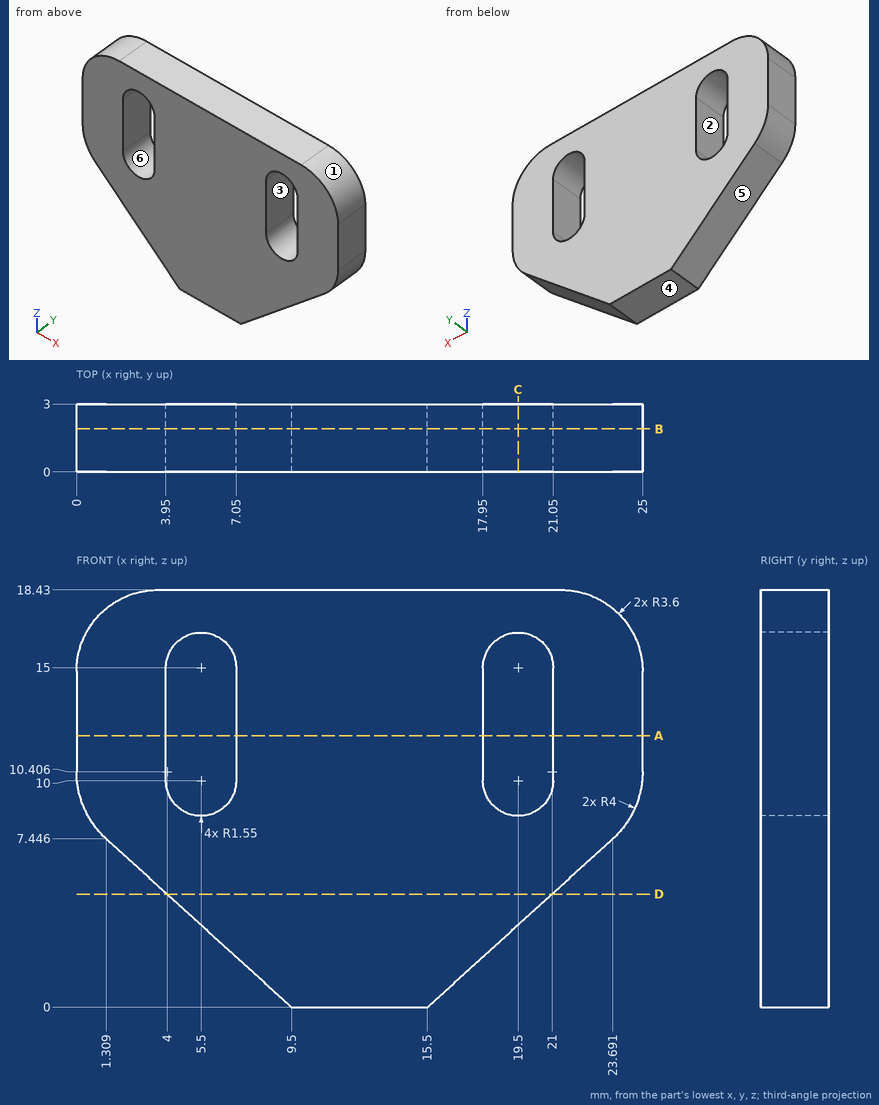
Job drawing, mm, ordinate dimensions from the low corner. One solid piece. A direction names the side the tool comes from. Give positions to 0.01 mm unless a question says otherwise; leave off trailing zeros. Loops run counter-clockwise (first coordinate to the right, second up) from the corner with the lowest first, then second, coordinate; pieces in that order, holes last. Notation, with made-up numbers: M -34.5,-31.5 L -11.5,-31.5 A17 cw -11.5,-11.5 Z; hole C -29.5,5.5 d2. An arc over 180 degrees is marked long. Put each result on its own line as item: value. Start each with the question number.
1) Flat gauge pins, fed straight in: pin 1 (8 mm diameter, centred on x = 20.5, z = 13, fed in from +Y); pin 2 (1 mm diameter, centred on y = 1, z = 16, fed in from -X). Where does each tip first touch, or does it go through?
2) Saw through at A-A (z = 12). List the corners of the cut face in (x, y), then the cut area to 3 significant figures.
3) Saw through at C-C (x = 19.5). List the corners of the cut face in (y, z).
4) Saw through at B-B (y = 1.9). List the corners of the cut face in (x, z), then the cut area to 3 significant figures.
5) Pull direction Z, two halves, no side cores. Call the marked faces 1, 2, 3 and 4: +Z half, -Z half, draft (parallel to the pull), parting line (faces both ways), or undercut.
6) Saw through at D-D (z = 5). List the corners of the cut face in (x, y), then the cut area to 3 significant figures.
7) 3-axis set-ups, long thin cutter, end or side, ignore diameter. For the marked faces 5 and 6: which of +Z, -Z, +X, -X, +Y, -Y reach the whole face in a straight line?
8) Probe probe 1 along X at (y, z) = (2.6, 11); probe 2 along X at (y, z) = (1.5, 9.75); probe 3 along Z at (x, y) = (19.75, 0.95) (1 decimal). List the from-to ranges inside material, lowest first.
Numbers:
1. pin 1: y = 3
1. pin 2: x = 0.06
2. outline: M 0,0 L 3.95,0 L 3.95,3 L 0,3 Z; M 7.05,0 L 17.95,0 L 17.95,3 L 7.05,3 Z; M 21.05,0 L 25,0 L 25,3 L 21.05,3 Z
2. area: 56.4 mm^2
3. outline: M 0,3.64 L 3,3.64 L 3,8.45 L 0,8.45 Z; M 0,16.55 L 3,16.55 L 3,18.43 L 0,18.43 Z
4. outline: M 0,10.41 A4 ccw 1.31,7.45 L 9.5,0 L 15.5,0 L 23.69,7.45 A4 ccw 25,10.41 L 25,14.83 A3.6 ccw 21.4,18.43 L 3.6,18.43 A3.6 ccw 0,14.83 Z; hole M 3.95,10 A1.55 ccw 7.05,10 L 7.05,15 A1.55 ccw 3.95,15 Z; hole M 17.95,10 A1.55 ccw 21.05,10 L 21.05,15 A1.55 ccw 17.95,15 Z
4. area: 326 mm^2
5. face 1: +Z half
5. face 2: undercut
5. face 3: undercut
5. face 4: -Z half
6. outline: M 4,0 L 21,0 L 21,3 L 4,3 Z
6. area: 51.0 mm^2
7. face 5: -Z, -X, +Y, -Y
7. face 6: +Y, -Y
8. probe 1: 0 to 3.95, 7.05 to 17.95, 21.05 to 25
8. probe 2: 0.05 to 3.97, 7.03 to 17.97, 21.03 to 24.95
8. probe 3: 3.9 to 8.5, 16.5 to 18.4
